Autodesk Inventor part; units mm, degrees
ref_plane "YZ Plane" through (0, 0, 0) normal (1, 0, 0) x (0, 1, 0)
ref_plane "XZ Plane" through (0, 0, 0) normal (0, 1, 0) x (-1, 0, 0)
ref_plane "XY Plane" through (0, 0, 0) normal (0, 0, 1) x (1, 0, 0)
sketch "Sketch1" plane through (0, 0, 0) normal (0, 1, 0) x (-1, 0, 0)
  circle A0 centre (0, 0) radius 1.5875
  line L0 (0, 0) -> (22.8671, 0) construction
  circle A1 centre (-49.53, 0) radius 1.5875
  circle A2 centre (-49.53, 0) radius 2.5
  line L1 (-24.765, 0) -> (-24.765, 33.4897) construction
  line L2 (0, 0) -> (0, -6.322) construction
  line L3 (-49.53, 0) -> (-44.53, 0) construction
  circle A3 centre (0, 0) radius 2.5
  dimension "d0" = 3.175
  dimension "d2" = 49.53
  dimension "d3" = 3.175
  dimension "d4" = 5
  dimension "d11" = 5
extrude "Extrusion1" add sketch "Sketch1" along normal blind 3
sketch "Sketch2" plane through (49.53, 0, 0) normal (0, -1, 0) x (1, 0, 0)
  line L0 (1, -2.2) -> (1, -5.2)
  line L1 (-1, -7.2) -> (-48.53, -7.2)
  line L2 (-50.53, -5.2) -> (-50.53, -2.2)
  line L3 (-48.53, -2.2) -> (-48.53, -4.2)
  line L4 (-47.53, -5.2) -> (-2, -5.2)
  line L5 (-1, -4.2) -> (-1, -2.2)
  line L6 (0, 0) -> (0, -7.7115) construction
  line L7 (1, -2.2) -> (-1, -2.2)
  line L8 (-49.53, 0) -> (-49.53, -7.2415) construction
  line L9 (-48.53, -2.2) -> (-50.53, -2.2)
  arc A0 (-48.53, -4.2) -> (-47.53, -5.2) centre (-47.53, -4.2) ccw
  arc A1 (-2, -5.2) -> (-1, -4.2) centre (-2, -4.2) ccw
  arc A2 (-50.53, -5.2) -> (-48.53, -7.2) centre (-48.53, -5.2) ccw
  arc A3 (-1, -7.2) -> (1, -5.2) centre (-1, -5.2) ccw
  point P0 (1, -7.2)
  point P1 (0, -2.2)
  point P2 (-49.53, -2.2)
  dimension "d14" = 5
  dimension "d15" = 2.2
  dimension "d16" = 2
  dimension "d17" = 2
  dimension "d18" = 2.2
  dimension "d19" = 1
  dimension "d20" = 2
extrude "Extrusion2" add sketch "Sketch2" against normal blind 3
sketch "Sketch3" plane through (48.53, 0, -7.2) normal (0, 0, -1) x (-1, 0, 0)
  arc A0 (20.5268, 1.5) -> (21.6698, 1.5) centre (21.0983, 1.5) ccw
  line L0 (47.53, 0) -> (0, 0) construction
  line L1 (21.0983, 0) -> (21.0983, 3) construction
  line L2 (0, 3) -> (47.53, 3)
  line L3 (-2, 0) -> (-2, 3)
  line L4 (21.6698, 1.5) -> (21.6698, 2.135)
  line L5 (21.6698, 2.135) -> (22.6698, 2.135)
  line L6 (22.6698, 2.135) -> (22.6698, 3)
  line L7 (20.5268, 1.5) -> (20.5268, 2.135)
  line L8 (20.5268, 2.135) -> (19.5268, 2.135)
  line L9 (19.5268, 2.135) -> (19.5268, 3)
  line L10 (21.0983, 1.5) -> (22.315, 1.5) construction
  line L11 (22.6698, 3) -> (19.5268, 3)
  point P0 (48.53, 0)
  point P1 (46.53, 3)
  point P2 (1, 3)
  dimension "d23" = 1.143
  dimension "d26" = 23.0983
  dimension "d27" = 1
  dimension "d28" = 1
  dimension "d29" = 0.635
  dimension "d30" = 0.635
  dimension "d31" = 1.5
extrude "Extrusion3" add sketch "Sketch3" along normal blind 5
pattern_linear "Rectangular Pattern1" count 2 spacing 23.241 along (1, 0, 0) of "Extrusion3"
sketch "Sketch4" plane through (49.1012, 3, -7.2) normal (0, 1, 0) x (1, 0, 0)
  arc A0 (0, -3.143) -> (3.143, 0) centre (0, 0) ccw
  line L0 (3.143, 0) -> (0, 0)
  line L1 (0, 0) -> (0, -3.143)
  point P0 (-49.1012, -7.2)
extrude "Extrusion4" add sketch "Sketch4" against normal blind 2.135
pattern_linear "Rectangular Pattern2" count 2 spacing 5.334 along (-1, 0, 0) of "Extrusion3"
pattern_linear "Rectangular Pattern3" count 2 spacing 28.575 along (-1, 0, 0) of "Extrusion3"
sketch "Sketch6" plane through (-2.7148, 3, -7.2) normal (0, 1, 0) x (1, 0, 0)
  arc A0 (0, 0) -> (3.143, -3.143) centre (3.143, 0) ccw
  line L0 (3.143, -3.143) -> (3.143, 0)
  line L1 (3.143, 0) -> (0, 0)
  point P0 (2.7148, -7.2)
extrude "Extrusion5" add sketch "Sketch6" against normal blind 2.135
sketch "Sketch7" plane through (52.2442, 3, -12.2) normal (0, 0, -1) x (-1, 0, 0)
  line L0 (2.143, -1.5) -> (2.143, -0.865) construction
  line L1 (2.143, -0.865) -> (3.143, -0.865) construction
  line L2 (3.143, -0.865) -> (3.143, 0) construction
  line L3 (3.143, 0) -> (0, 0) construction
  line L4 (0, 0) -> (0, -0.865) construction
  line L5 (0, -0.865) -> (1, -0.865) construction
  line L6 (1, -0.865) -> (1, -1.5) construction
  arc A0 (1, -1.5) -> (2.143, -1.5) centre (1.5715, -1.5) ccw construction
  line L7 (0, -0.865) -> (0, 0)
  line L8 (0, 0) -> (3.143, 0)
  line L9 (3.143, 0) -> (3.143, -0.865)
  arc A1 (0, -0.865) -> (3.143, -0.865) centre (1.5715, -0.865) ccw
  line L10 (3.143, -0.865) -> (0, -0.865) construction
  line L11 (3.143, -0.865) -> (3.143, 0) construction
  point P0 (52.2442, -3)
extrude "Extrusion6" add sketch "Sketch7" against normal blind 2
pattern_linear "Rectangular Pattern4" count 2 spacing 23.241 along (-1, 0, 0) of "Extrusion6"
pattern_linear "Rectangular Pattern5" count 2 spacing 28.575 along (-1, 0, 0) of "Extrusion6"
pattern_linear "Rectangular Pattern6" count 2 spacing 51.816 along (-1, 0, 0) of "Extrusion6"
sketch "Sketch8" plane through (48.53, 0, -7.2) normal (0, 0, -1) x (-1, 0, 0)
  line L0 (-4.8097, 14.9523) -> (52.3403, 14.9523) construction
  line L1 (52.3403, 14.9523) -> (52.3403, 4.9523) construction
  line L2 (52.3403, 4.9523) -> (-4.8097, 4.9523) construction
  line L3 (-4.8097, 4.9523) -> (-4.8097, 14.9523) construction
  line L4 (-4.6827, 26.2305) -> (23.6383, 26.2305) construction
  line L5 (23.6383, 26.2305) -> (23.6383, 17.1827) construction
  line L6 (23.6383, 17.1827) -> (-4.6827, 17.1827) construction
  line L7 (-4.6827, 17.1827) -> (-4.6827, 26.2305) construction
  line L8 (52.2133, 26.2305) -> (23.8923, 26.2305) construction
  line L9 (23.8923, 26.2305) -> (23.8923, 17.1827) construction
  line L10 (23.8923, 17.1827) -> (52.2133, 17.1827) construction
  line L11 (52.2133, 17.1827) -> (52.2133, 26.2305) construction
  circle A0 centre (-2.1427, 14.9523) radius 0.635
  circle A1 centre (21.0983, 14.9523) radius 0.635
  circle A2 centre (26.4323, 14.9523) radius 0.635
  circle A3 centre (49.6733, 14.9523) radius 0.635
  arc A4 (-2.7142, 1.5) -> (-1.5712, 1.5) centre (-2.1427, 1.5) ccw
  line L12 (-2.1427, 1.5) -> (-2.1427, 11.5483) construction
  arc A5 (20.5268, 1.5) -> (21.6698, 1.5) centre (21.0983, 1.5) ccw construction
  arc A6 (25.8608, 1.5) -> (27.0038, 1.5) centre (26.4323, 1.5) ccw construction
  arc A7 (49.1018, 1.5) -> (50.2448, 1.5) centre (49.6733, 1.5) ccw construction
  line L13 (21.0983, 1.5) -> (21.0983, 9.9523) construction
  line L14 (26.4323, 1.5) -> (26.4323, 9.0967) construction
  line L15 (49.6733, 1.5) -> (49.6733, 9.9523) construction
  line L16 (24.8608, 2.135) -> (24.8608, 3) construction
  line L17 (22.6698, 3) -> (24.8608, 3) construction
  line L18 (22.6698, 3) -> (22.6698, 2.135) construction
  line L19 (22.6698, 2.135) -> (21.6698, 2.135) construction
  line L20 (21.6698, 2.135) -> (21.6698, 1.5) construction
  arc A8 (20.5268, 1.5) -> (21.6698, 1.5) centre (21.0983, 1.5) ccw construction
  line L21 (20.5268, 1.5) -> (20.5268, 2.135) construction
  line L22 (20.5268, 2.135) -> (19.5268, 2.135) construction
  line L23 (19.5268, 2.135) -> (19.5268, 3) construction
  line L24 (0, 3) -> (19.5268, 3) construction
  line L25 (0, 0) -> (0, 3) construction
  line L26 (47.53, 0) -> (0, 0) construction
  line L27 (47.53, 0) -> (47.53, 3) construction
  line L28 (28.0038, 3) -> (47.53, 3) construction
  line L29 (28.0038, 3) -> (28.0038, 2.135) construction
  line L30 (28.0038, 2.135) -> (27.0038, 2.135) construction
  line L31 (27.0038, 2.135) -> (27.0038, 1.5) construction
  arc A9 (25.8608, 1.5) -> (27.0038, 1.5) centre (26.4323, 1.5) ccw construction
  line L32 (25.8608, 1.5) -> (25.8608, 2.135) construction
  line L33 (25.8608, 2.135) -> (24.8608, 2.135) construction
  line L34 (47.53, 0) -> (0, 0) construction
  line L35 (23.765, 0) -> (23.765, 9.6631) construction
  point P0 (48.53, 0)
  dimension "d57" = 57.15
  dimension "d58" = 10
  dimension "d59" = 28.321
  dimension "d60" = 0.127
  dimension "d61" = 28.321
  dimension "d62" = 0.254
  dimension "d63" = 0.127
  dimension "d64" = 1.27
  dimension "d65" = 2.54
  dimension "d66" = 1.27
  dimension "d67" = 2.54
  dimension "d68" = 1.27
  dimension "d69" = 1.27
  dimension "d70" = 2.54
  dimension "d71" = 2.54
  dimension "d72" = 23.241
  dimension "d73" = 5.334
  dimension "d74" = 23.241
  dimension "d75" = 2.6673
  dimension "d76" = 2.6667
properties part number "HDMIPluginModuleHolder01"
Geometry check sheet. Reference: the model listing, model coordinates, mm. A direction names the side the tool comes from. Round coordinates to 2 decimals unless told otherwise and drop trailing zeros. Write each loop counter-clockwise with the first axis right and the second up, starting at its lowest first coordinate (ties: lowest second). Pieces come first, ordered by that corner, then holes. Notation, with made-up numbers: (-33.75, -3.75) -> (-5.75, -3.75) arc R32 ccw to (-5.75, 32.25) -> close; hole circle Ø7 at (-33, 65.25). An arc over 180 degrees is marked (long way). One line per item, written item: value. Start each with the question number.
(1) Access from +Z, -Z, +X, -X, +Y, -Y to the whole of each face (thin tool, end or side, straight path). Record for faces 1 (the flat face through (29.003, 2.6, -9.7)), 2 (the flat face through (52, 2.135, -9)), 3 (the cylindrical face through (51.77, 1.95, -5.54)), 4 (the flat face through (-1, 1, -3)), 5 (the flat face through (28.5, 2.135, -8.7)).
(2) Go/stop test with flat-tipped pins: pin 1 Ø0.7 at (y, z) = (2, -9) entering from +X; pin 2 Ø1.5 at (x, y) = (45, 1) entering from +Z. Record where each tip stops, or that it passes through.
(3) Cross-section at C-C, the plane x = 14.5. Record the cut outline in (y, z), and give its area (3 significant figures).
(4) Cross-section at A-A, the plane z = -9. Give the number of separate pieces and of enclosed holes in the cut face, and give its area (3 significant figures).
(5) Cross-section at B-B, the plane z = 0. Record the cut outline in (x, y), and give its area (4 significant figures).
(6) Scan lines: line 1 (Z direction, x = 49.53, y = 1.3); line 2 (Z direction, x = 21.5, y = 1.25); line 3 (X direction, y = 1, z = -9). Record each from-to range of solid material in increasing order. Write a range as [from, to].
Answer:
1. face 1: -Z, +Y, -Y
1. face 2: +X, -Y
1. face 3: +X, +Y, -Y
1. face 4: -X, -Y
1. face 5: -Y
2. pin 1: x = 52.24
2. pin 2: z = -5.2
3. outline: (0, -7.2) -> (3, -7.2) -> (3, -5.2) -> (0, -5.2) -> close
3. area: 6.00 mm²
4. separate pieces: 4
4. enclosed holes: 0
4. area: 15.8 mm²
5. outline: (-2.5, 0) -> (-1.59, 0) -> (-1.59, 3) -> (-2.5, 3) -> close; (1.59, 0) -> (2.5, 0) -> (2.5, 3) -> (1.59, 3) -> close; (47.03, 0) -> (47.94, 0) -> (47.94, 3) -> (47.03, 3) -> close; (51.12, 0) -> (52.03, 0) -> (52.03, 3) -> (51.12, 3) -> close
5. area: 10.95 mm²
6. line 1: [-12.2, -10.2], [-7.2, -1.59], [1.59, 2.5]
6. line 2: [-12.2, -10.2], [-7.2, -5.2]
6. line 3: [-1.42, -0.87], [21.82, 22.37], [27.15, 27.71], [50.4, 50.95]
